Here's how the part is built. I have some questions about the finished solid (model axes, mm). Coordinates: 2 decimals unless noted, no trailing zeros. Write each loop counter-clockwise with the first axis right and the second up, starting at its lowest first coordinate (ties: lowest second). Pieces come first, ordered by that corner, then holes. Notation, with made-up numbers: (59.5, 12) - (97.5, 12) arc R29 cw to (97.5, 46) - close; hole circle Ø3 at (-18, -18.75). An arc over 180 degrees is marked (long way). Answer in a Markdown table with one row per item. Add a question column.
Item 1: Imagine slicing it at A-A (z = -9). Please give me the cut outline in (x, y), plus the area to 3 significant figures.
Item 2: If I drill on probe 1 along Y at (x, z) = (24.5, -2.25); probe 2 along Y at (x, z) = (45, -9.25); probe 3 along X at (y, z) = (35, -7), over which ranges is the centre line in solid material (lowest first)? Write a range as from..to.
Item 3: I'm going to push a flat-ended pin straight in: pin 1 (3 mm diameter, centred on y = 40, z = -4.5, fed in from +X). Where does the tip first touch, or does it pass through?
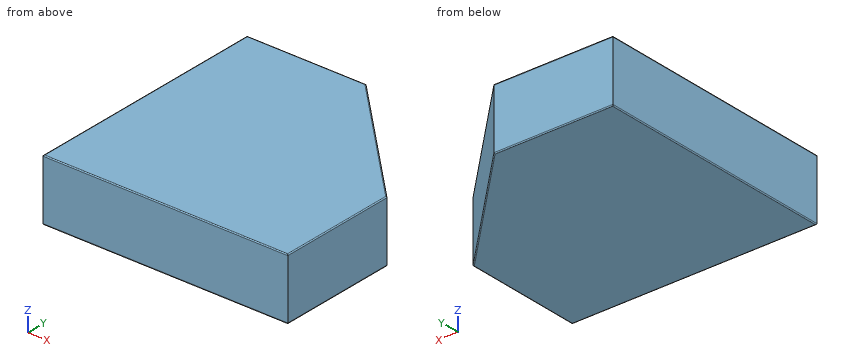
from build123d import *

# Parameters (mm, degrees)
F1_DEPTH = 12.5
F2_R     = 0.2


with BuildPart() as f1:
    # F0 (on Top) → F1 (new body)
    with BuildSketch(Plane.XY):
        Polygon((0, 50), (0, 0), (50, 0), (50, 24.3), (24.3, 50), align=None)
    extrude(amount=-F1_DEPTH)

    # F2
    f2_edges = [f1.edges().sort_by_distance(p)[0] for p in [
        (12.15, 50, 0),
        (0, 25, 0),
        (25, 0, 0),
        (50, 12.15, 0),
        (37.15, 37.15, 0),
        (12.15, 50, -12.5),
        (0, 25, -12.5),
        (25, 0, -12.5),
        (50, 12.15, -12.5),
        (37.15, 37.15, -12.5),
    ]]
    fillet(f2_edges, radius=F2_R)


solid = f1.part
Here are the results:
| question | item | result |
|---|---|---|
| 1 | outline | (0, 0) - (50, 0) - (50, 24.3) - (24.3, 50) - (0, 50) - close |
| 1 | area | 2,170 mm2 |
| 2 | probe 1 | y = 0..49.8 |
| 2 | probe 2 | y = 0..29.3 |
| 2 | probe 3 | x = 0..39.3 |
| 3 | pin 1 | stops at x = 35.8 |
